from build123d import *

# Parameters (mm, degrees)
SKETCH1_W                         = 12.7
SKETCH1_H                         = 50.8
BASE_EXTRUDE_DEPTH                = 6.35
SKETCH6_W                         = 12.7
SKETCH6_H                         = 6.35
ARCH_BASE_EXTRUDE_DEPTH           = 10.16
ARCH_EXTRUDE_DEPTH                = 6.35
SKETCH3_R                         = 3.175
ARCH_HOLE_CUT_DEPTH               = 6.35
SKETCH4_W                         = 25.4
SKETCH4_H                         = 6.35
TAB_EXTRUDE_DEPTH                 = 63.5
SKETCH5_W                         = 3.175
SKETCH5_H                         = 25.4
SQUARE_SLIDE_GUIDES_EXTRUDE_DEPTH = 19.05
SKETCH14_R                        = 3.175
CUT_EXTRUDE3_DEPTH                = 13.97


with BuildPart() as part:
    # Sketch1 → Base Extrude (new body)
    with BuildSketch(Plane(origin=(0, 0, 0), x_dir=(1, 0, 0), z_dir=(0, 1, 0))):
        with Locations((-6.35, 25.4)):
            Rectangle(SKETCH1_W, SKETCH1_H)
    extrude(amount=BASE_EXTRUDE_DEPTH)

    # Sketch6 → Arch Base Extrude (add)
    with BuildSketch(Plane(origin=(0, 6.35, 0), x_dir=(1, 0, 0), z_dir=(0, 1, 0))):
        with Locations((-6.35, 3.175)):
            Rectangle(SKETCH6_W, SKETCH6_H)
    arch_base_extrude = extrude(amount=ARCH_BASE_EXTRUDE_DEPTH)

    # Mirror Arch Base: Arch Base Extrude across plane
    add(arch_base_extrude.mirror(Plane.XY.offset(-25.4)))

    # Sketch2 → Arch Extrude (add)
    with BuildSketch(Plane.XY):
        with BuildLine():
            Line((-12.7, 16.51), (0, 16.51))
            ThreePointArc((0, 16.51), (-6.35, 22.86), (-12.7, 16.51))
        make_face()
    arch_extrude = extrude(amount=-ARCH_EXTRUDE_DEPTH)

    # Sketch3 → Arch Hole Cut (cut)
    with BuildSketch(Plane.XY):
        with Locations((-6.35, 16.51)):
            Circle(SKETCH3_R)
    arch_hole_cut = extrude(amount=-ARCH_HOLE_CUT_DEPTH, mode=Mode.SUBTRACT)

    # Mirror Arch and Hole: Arch Extrude, Arch Hole Cut across plane
    add(arch_extrude.mirror(Plane.XY.offset(-25.4)))
    add(arch_hole_cut.mirror(Plane.XY.offset(-25.4)), mode=Mode.SUBTRACT)

    # Sketch4 → Tab Extrude (add)
    with BuildSketch(Plane(origin=(0, 0, 0), x_dir=(0, 0, -1), z_dir=(1, 0, 0))):
        with Locations((25.4, 3.175)):
            Rectangle(SKETCH4_W, SKETCH4_H)
    extrude(amount=TAB_EXTRUDE_DEPTH)

    # Sketch5 → Square Slide Guides Extrude (add)
    with BuildSketch(Plane(origin=(0, 6.35, 0), x_dir=(1, 0, 0), z_dir=(0, 1, 0))):
        with Locations((42.2275, 25.4)):
            Rectangle(SKETCH5_W, SKETCH5_H)
        with Locations((53.0225, 25.4)):
            Rectangle(SKETCH5_W, SKETCH5_H)
    extrude(amount=SQUARE_SLIDE_GUIDES_EXTRUDE_DEPTH)

    # Sketch14 → Cut-Extrude3 (cut)
    with BuildSketch(Plane(origin=(54.61, 0, 0), x_dir=(0, 0, -1), z_dir=(1, 0, 0))):
        with Locations((25.4, 16.51)):
            Circle(SKETCH14_R)
    extrude(amount=-CUT_EXTRUDE3_DEPTH, mode=Mode.SUBTRACT)


solid = part.part
Here's how the part is built. I have some questions about the finished solid (model axes, mm). A direction names the side the tool comes from. Coordinates: 2 decimals unless noted, no trailing zeros. Loops run counter-clockwise (first coordinate to the right, second up) from the corner with the lowest first, then second, coordinate; pieces in that order, holes last. Notation, with made-up numbers: (-9.5, -25) -> (-2.5, -25) arc R16 cw to (-2.5, -9) -> close; hole circle Ø2 at (-24, -3). An arc over 180 degrees is marked (long way). Use one line per item in the form item = value. Start each with the question number.
(1) On a 3-axis mill with a long thin cutter (end or side, diameter ignored), from which of +Z, -Z, +X, -X, +Y, -Y can I reach the whole of each face in a straight line? I mean faces 1 (the face through (14, 6.35, -26)), 2 (the face through (0, 6, -5)), 3 (the face through (-6, 13, -44.45)), 4 (the face through (34, 5, -38.1)), 5 (the face through (43.815, 14, -22)). Say none if no direction works.
(2) If we section it at B-B (y = 10): Please give me the cut outline in (x, z) (3 decimals), then the cut area to 3 significant figures.
(3) If we section it at D-D (z = -25.4): Please give me the cut outline in (x, y) (3 decimals), then the cut area to 3 significant figures.
(4) If we section it at C-C (z = -45.5): Please give me the cut outline in (x, y) (3 decimals).
(5) We'd pull the mould along X, two halves only. Please class faces 6 (the face through (34, 5, -12.7)), 7 (the face through (0, 6, -46)), 8 (the face through (51.435, 14, -22)): pulls with the +X half, pulls with the -X half, needs draft (parallel to the pull), parting line crosses it, or undercut.
(6) If we section it at A-A (x = -6.35): Please give me the cut outline in (y, z) (3 decimals).
(7) Please list where these lines run through material, in increasing order: line 1 along Y through (x, z) = (42.4, -25.4) (3 decimals); line 2 along Y through (x, z) = (-6.35, -47.25) (3 decimals); line 3 along X through (y, z) = (20.5, -18) (3 decimals).
(8) Will these pins go through, and if not, where does the flat tip stop? pin 1 (14 mm diameter, centred on x = -9.5, y = 16, fed in from +Z); pin 2 (3 mm diameter, centred on x = 51.5, y = 20, fed in from -Z); pin 3 (7 mm diameter, centred on x = 60.5, z = -27.5, fed in from +Y); pin 4 (1.5 mm diameter, centred on y = 22.5, z = -25, fed in from -X).
Verdict:
q1.face_1 = -X, +Y
q1.face_2 = +Z, +X, +Y, -Y
q1.face_3 = +X, -X, +Y
q1.face_4 = -Z, +X, +Y, -Y
q1.face_5 = +Z, -Z, +Y
q2.outline = (-12.7, -50.8) -> (0, -50.8) -> (0, -44.45) -> (-12.7, -44.45) -> close; (-12.7, -6.35) -> (0, -6.35) -> (0, 0) -> (-12.7, 0) -> close; (40.64, -38.1) -> (43.815, -38.1) -> (43.815, -12.7) -> (40.64, -12.7) -> close; (51.435, -38.1) -> (54.61, -38.1) -> (54.61, -12.7) -> (51.435, -12.7) -> close
q2.area = 323 mm²
q3.outline = (-12.7, 0) -> (63.5, 0) -> (63.5, 6.35) -> (54.61, 6.35) -> (54.61, 13.335) -> (51.435, 13.335) -> (51.435, 6.35) -> (43.815, 6.35) -> (43.815, 13.335) -> (40.64, 13.335) -> (40.64, 6.35) -> (-12.7, 6.35) -> close; (40.64, 19.685) -> (43.815, 19.685) -> (43.815, 25.4) -> (40.64, 25.4) -> close; (51.435, 19.685) -> (54.61, 19.685) -> (54.61, 25.4) -> (51.435, 25.4) -> close
q3.area = 565 mm²
q4.outline = (-12.7, 0) -> (0, 0) -> (0, 16.51) arc R6.35 ccw to (-12.7, 16.51) -> close; hole circle Ø6.35 at (-6.35, 16.51)
q5.face_6 = needs draft
q5.face_7 = pulls with the +X half
q5.face_8 = undercut
q6.outline = (0, -50.8) -> (13.335, -50.8) -> (13.335, -44.45) -> (6.35, -44.45) -> (6.35, -6.35) -> (13.335, -6.35) -> (13.335, 0) -> (0, 0) -> close; (19.685, -50.8) -> (22.86, -50.8) -> (22.86, -44.45) -> (19.685, -44.45) -> close; (19.685, -6.35) -> (22.86, -6.35) -> (22.86, 0) -> (19.685, 0) -> close
q7.line_1 = 0 to 13.335, 19.685 to 25.4
q7.line_2 = 0 to 13.335, 19.685 to 22.86
q7.line_3 = 40.64 to 43.815, 51.435 to 54.61
q8.pin_1 = 0
q8.pin_2 = -38.1
q8.pin_3 = 6.35
q8.pin_4 = 40.64
